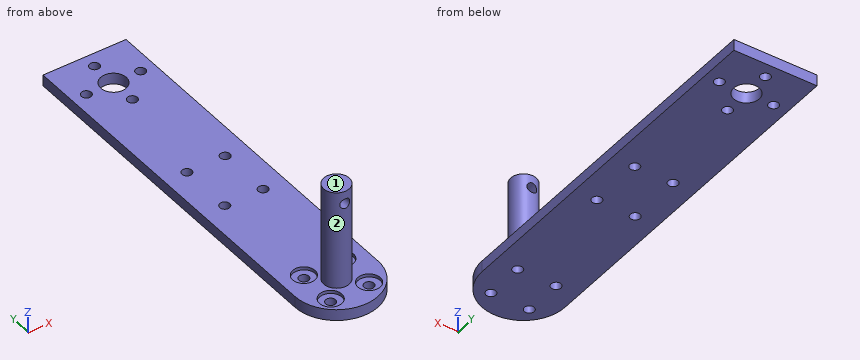
from build123d import *

# Parameters (mm, degrees)
SKETCH1_R                           = 1.55
SKETCH1_R_2                         = 4
BOSS_EXTRUDE1_DEPTH                 = 3.5
SKETCH2_R                           = 4
BOSS_EXTRUDE2_DEPTH                 = 31
SKETCH3_R                           = 3.5
CUT_EXTRUDE1_DEPTH                  = 1
CUT_EXTRUDE2_REACH                  = 120.862
CUT_EXTRUDE2_END_RADIUS             = 4
SKETCH4_R                           = 1.55
CUT_EXTRUDE2_DIRECTION_2_REACH      = 120.862
CUT_EXTRUDE2_DIRECTION_2_END_RADIUS = 4


with BuildPart() as part:
    # Sketch1 → Boss-Extrude1 (new body)
    with BuildSketch(Plane.XY):
        with BuildLine():
            Line((13, 0), (13, 113))
            Line((13, 113), (-13, 113))
            Line((-13, 113), (-13, 0))
            ThreePointArc((-13, 0), (0, -13), (13, 0))
        make_face()
        with Locations((6.01040764, 6.01040764)):
            Circle(SKETCH1_R, mode=Mode.SUBTRACT)
        with Locations((6.01040764, -6.01040764)):
            Circle(SKETCH1_R, mode=Mode.SUBTRACT)
        with Locations((-6.01040764, -6.01040764)):
            Circle(SKETCH1_R, mode=Mode.SUBTRACT)
        with Locations((-6.01040764, 6.01040764)):
            Circle(SKETCH1_R, mode=Mode.SUBTRACT)
        with Locations((0, 100)):
            Circle(SKETCH1_R_2, mode=Mode.SUBTRACT)
        with Locations((0, 108.5)):
            Circle(SKETCH1_R, mode=Mode.SUBTRACT)
        with Locations((8.5, 100)):
            Circle(SKETCH1_R, mode=Mode.SUBTRACT)
        with Locations((0, 91.5)):
            Circle(SKETCH1_R, mode=Mode.SUBTRACT)
        with Locations((-8.5, 100)):
            Circle(SKETCH1_R, mode=Mode.SUBTRACT)
        with Locations((6, 58.5)):
            Circle(SKETCH1_R, mode=Mode.SUBTRACT)
        with Locations((6, 41.5)):
            Circle(SKETCH1_R, mode=Mode.SUBTRACT)
        with Locations(Location((-6, 58.5, 0), (0, 0, 180))):
            Circle(SKETCH1_R, mode=Mode.SUBTRACT)
        with Locations(Location((-6, 41.5, 0), (0, 0, 180))):
            Circle(SKETCH1_R, mode=Mode.SUBTRACT)
    extrude(amount=BOSS_EXTRUDE1_DEPTH)

    # Sketch2 → Boss-Extrude2 (add)
    with BuildSketch(Plane.XY.offset(3.5)):
        with Locations(Location((0, 0, 0), (0, 0, 180))):
            Circle(SKETCH2_R)
    extrude(amount=BOSS_EXTRUDE2_DEPTH)

    # Sketch3 → Cut-Extrude1 (cut)
    with BuildSketch(Plane.XY.offset(3.5)):
        with Locations((-6.01040764, 6.01040764)):
            Circle(SKETCH3_R)
        with Locations((6.01040764, 6.01040764)):
            Circle(SKETCH3_R)
        with Locations((6.01040764, -6.01040764)):
            Circle(SKETCH3_R)
        with Locations((-6.01040764, -6.01040764)):
            Circle(SKETCH3_R)
    extrude(amount=-CUT_EXTRUDE1_DEPTH, mode=Mode.SUBTRACT)

    # Cut-Extrude2: up to this cylinder (the profile starts inside it)
    cut_extrude2_end = Plane(origin=(0, 0, 30.5), z_dir=(0, 0, -1)) * Cylinder(CUT_EXTRUDE2_END_RADIUS, 250.724, mode=Mode.PRIVATE)
    # Sketch4 → Cut-Extrude2 (cut, up to the surface)
    with BuildSketch(Plane(origin=(0, 0, 0), x_dir=(0, 0, -1), z_dir=(0, -1, 0)), mode=Mode.PRIVATE) as cut_extrude2_sk1:
        with Locations((-30.5, 0)):
            Circle(SKETCH4_R)
    cut_extrude2_tool1 = extrude(cut_extrude2_sk1.sketch, amount=-CUT_EXTRUDE2_REACH, mode=Mode.PRIVATE) & cut_extrude2_end
    add(cut_extrude2_tool1.solids().sort_by_distance((0, 0, 30.5))[0], mode=Mode.SUBTRACT)

    # Cut-Extrude2 direction 2: up to this cylinder (the profile starts inside it)
    cut_extrude2_direction_2_end = Plane(origin=(0, 0, 30.5), z_dir=(0, 0, -1)) * Cylinder(CUT_EXTRUDE2_DIRECTION_2_END_RADIUS, 250.724, mode=Mode.PRIVATE)
    # Sketch4 → Cut-Extrude2 direction 2 (cut, up to the surface)
    with BuildSketch(Plane(origin=(0, 0, 0), x_dir=(0, 0, -1), z_dir=(0, -1, 0)), mode=Mode.PRIVATE) as cut_extrude2_direction_2_sk1:
        with Locations((-30.5, 0)):
            Circle(SKETCH4_R)
    cut_extrude2_direction_2_tool1 = extrude(cut_extrude2_direction_2_sk1.sketch, amount=CUT_EXTRUDE2_DIRECTION_2_REACH, mode=Mode.PRIVATE) & cut_extrude2_direction_2_end
    add(cut_extrude2_direction_2_tool1.solids().sort_by_distance((0, 0, 30.5))[0], mode=Mode.SUBTRACT)


solid = part.part
CAD build for the part. Positions are in the model's coordinates, mm. Face numbers are marked on the shaded views. A direction names the side the tool comes from. Round coordinates to 2 decimals unless told otherwise and drop trailing zeros. Write each loop counter-clockwise with the first axis right and the second up, starting at its lowest first coordinate (ties: lowest second). Pieces come first, ordered by that corner, then holes. Notation, with made-up numbers: M 65.5,46.5 L 101.5,46.5 A24 cw 101.5,68.5 Z; hole C -4.5,15 d10. An arc over 180 degrees is marked long. Put each result on its own line as item: value. Start each with the question number.
1) Saw through at B-B, the plane y = 100. Write the cut outline in (x, z), and give its area (3 significant figures).
2) Pin check, flat tips, straight feed: pin 1 Ø1 at (x, z) = (2.5, 25.5) entering from +Y; pin 2 Ø5.5 at (x, y) = (-6.01, -6.01) entering from +Z; pin 3 Ø7.5 at (x, y) = (6, -5) entering from +Z; pin 4 Ø1.9 at (x, y) = (-6.01, -6.01) entering from +Z. Stop position of each tip, or through.
3) Drill centre lines: probe 1 along Y at (x, z) = (0, 1.8); probe 2 along Z at (x, y) = (2.5, 76.5); probe 3 along Y at (x, z) = (-3.25, 15). Where is each one in solid material? Low to high. Write a range as [from, to].
4) Saw through at A-A, the plane y = 58.5. Write the cut outline in (x, z), and give its area (3 significant figures).
5) Saw through at D-D, the plane y = 81. Write the cut outline in (x, z), and give its area (3 significant figures).
6) 3-axis set-ups, long thin cutter, end or side, ignore diameter. For the marked faces 1 and 2: which of +Z, -Z, +X, -X, +Y, -Y reach the whole face in a straight line?
7) Saw through at C-C, the plane z = 14. Write the cut outline in (x, y), and give its area (3 significant figures).
Resolved:
1. outline: M -13,0 L -10.05,0 L -10.05,3.5 L -13,3.5 Z; M -6.95,0 L -4,0 L -4,3.5 L -6.95,3.5 Z; M 4,0 L 6.95,0 L 6.95,3.5 L 4,3.5 Z; M 10.05,0 L 13,0 L 13,3.5 L 10.05,3.5 Z
1. area: 41.3 mm²
2. pin 1: y = 3.46
2. pin 2: z = 2.5
2. pin 3: z = 3.5
2. pin 4: through
3. probe 1: [-13, 89.95], [93.05, 96], [104, 106.95], [110.05, 113]
3. probe 2: [0, 3.5]
3. probe 3: [-2.33, 2.33]
4. outline: M -13,0 L -7.55,0 L -7.55,3.5 L -13,3.5 Z; M -4.45,0 L 4.45,0 L 4.45,3.5 L -4.45,3.5 Z; M 7.55,0 L 13,0 L 13,3.5 L 7.55,3.5 Z
4. area: 69.3 mm²
5. outline: M -13,0 L 13,0 L 13,3.5 L -13,3.5 Z
5. area: 91.0 mm²
6. face 1: +Z, +X, -X, +Y, -Y
6. face 2: +Z
7. outline: C 0,0 d8
7. area: 50.3 mm²
